Geometry check sheet. Reference: the model listing, model coordinates, mm. Round coordinates to 2 decimals unless told otherwise and drop trailing zeros. Loops run counter-clockwise (first coordinate to the right, second up) from the corner with the lowest first, then second, coordinate; pieces in that order, holes last. Notation, with made-up numbers: M 14.25,74 L 42.25,74 A28 cw 42.25,103 Z; hole C 3,57 d8. An arc over 180 degrees is marked long. Use one line per item in the form item = value. Start each with the question number.
1. Cross-section at C-C (z = 0.1). Record the boundary of the cut face in (x, y), then the cut area to 3 significant figures.
2. Cross-section at A-A (x = 1.5). Record the boundary of the cut face in (y, z).
3. Material ranges on line 1 (X direction, y = 0, z = 0.15); line 2 (X direction, y = 5.25, z = 0.05), recorded low to high.
4. Draft check along X on faces 1 (the flat face through (-7, -2, 0.2)), 2 (the flat face through (2, -7, 0.2)). Enter one of: pulls with the +X half, pulls with the -X half, needs draft (parallel to the pull), parting line crosses it, or undercut.
5. Cross-section at B-B (y = 1). Record the boundary of the cut face in (x, z).
6. Go/stop test with a flat-tipped pin: pin 1 (6 mm diameter, centred on x = 3.5, y = 3.5, fed in from +Z). Record where the tip stops, or that it passes through.
```python
from build123d import *
from build123d.topology import SkipClean

# Parameters (mm, degrees)
SKETCH1_R           = 7.5
SKETCH1_R_2         = 6.75
BOSS_EXTRUDE1_DEPTH = 0.2
BOSS_EXTRUDE3_DEPTH = 0.03


with BuildPart() as part:
    # Sketch1 → Boss-Extrude1 (new body)
    with BuildSketch(Plane.XY):
        Circle(SKETCH1_R)
        Circle(SKETCH1_R_2, mode=Mode.SUBTRACT)
    extrude(amount=BOSS_EXTRUDE1_DEPTH)

    # Sketch2 → Boss-Extrude3 (add)
    with SkipClean():  # the faces are left unmerged after this step: merging them gives an invalid solid
        with BuildSketch(Plane.XY.offset(0.2)):
            with BuildLine():
                Line((3.663064111, 6.544613152), (3.288027069, 5.89502994))
                ThreePointArc((3.288027069, 5.89502994), (3.375, 5.845671476), (3.46123215, 5.79502994))
                Line((3.46123215, 5.79502994), (3.836269192, 6.444613152))
                ThreePointArc((3.836269192, 6.444613152), (3.75, 6.495190528), (3.663064111, 6.544613152))
            make_face()
            with BuildLine():
                Line((-0.1, 7.499333304), (-0.1, 6.749259219))
                ThreePointArc((-0.1, 6.749259219), (0, 6.75), (0.1, 6.749259219))
                Line((0.1, 6.749259219), (0.1, 7.499333304))
                ThreePointArc((0.1, 7.499333304), (0, 7.5), (-0.1, 7.499333304))
            make_face()
            with BuildLine():
                Line((6.444613152, 3.836269192), (5.79502994, 3.46123215))
                ThreePointArc((5.79502994, 3.46123215), (5.845671476, 3.375), (5.89502994, 3.288027069))
                Line((5.89502994, 3.288027069), (6.544613152, 3.663064111))
                ThreePointArc((6.544613152, 3.663064111), (6.495190528, 3.75), (6.444613152, 3.836269192))
            make_face()
            with BuildLine():
                Line((7.499333304, 0.1), (6.749259219, 0.1))
                ThreePointArc((6.749259219, 0.1), (6.75, 0), (6.749259219, -0.1))
                Line((6.749259219, -0.1), (7.499333304, -0.1))
                ThreePointArc((7.499333304, -0.1), (7.5, 0), (7.499333304, 0.1))
            make_face()
            with BuildLine():
                Line((6.544613152, -3.663064111), (5.89502994, -3.288027069))
                ThreePointArc((5.89502994, -3.288027069), (5.845671476, -3.375), (5.79502994, -3.46123215))
                Line((5.79502994, -3.46123215), (6.444613152, -3.836269192))
                ThreePointArc((6.444613152, -3.836269192), (6.495190528, -3.75), (6.544613152, -3.663064111))
            make_face()
            with BuildLine():
                Line((3.836269192, -6.444613152), (3.46123215, -5.79502994))
                ThreePointArc((3.46123215, -5.79502994), (3.375, -5.845671476), (3.288027069, -5.89502994))
                Line((3.288027069, -5.89502994), (3.663064111, -6.544613152))
                ThreePointArc((3.663064111, -6.544613152), (3.75, -6.495190528), (3.836269192, -6.444613152))
            make_face()
            with BuildLine():
                Line((0.1, -7.499333304), (0.1, -6.749259219))
                ThreePointArc((0.1, -6.749259219), (0, -6.75), (-0.1, -6.749259219))
                Line((-0.1, -6.749259219), (-0.1, -7.499333304))
                ThreePointArc((-0.1, -7.499333304), (0, -7.5), (0.1, -7.499333304))
            make_face()
            with BuildLine():
                Line((-3.663064111, -6.544613152), (-3.288027069, -5.89502994))
                ThreePointArc((-3.288027069, -5.89502994), (-3.375, -5.845671476), (-3.46123215, -5.79502994))
                Line((-3.46123215, -5.79502994), (-3.836269192, -6.444613152))
                ThreePointArc((-3.836269192, -6.444613152), (-3.75, -6.495190528), (-3.663064111, -6.544613152))
            make_face()
            with BuildLine():
                Line((-6.444613152, -3.836269192), (-5.79502994, -3.46123215))
                ThreePointArc((-5.79502994, -3.46123215), (-5.845671476, -3.375), (-5.89502994, -3.288027069))
                Line((-5.89502994, -3.288027069), (-6.544613152, -3.663064111))
                ThreePointArc((-6.544613152, -3.663064111), (-6.495190528, -3.75), (-6.444613152, -3.836269192))
            make_face()
            with BuildLine():
                Line((-7.499333304, -0.1), (-6.749259219, -0.1))
                ThreePointArc((-6.749259219, -0.1), (-6.75, 0), (-6.749259219, 0.1))
                Line((-6.749259219, 0.1), (-7.499333304, 0.1))
                ThreePointArc((-7.499333304, 0.1), (-7.5, 0), (-7.499333304, -0.1))
            make_face()
            with BuildLine():
                Line((-6.544613152, 3.663064111), (-5.89502994, 3.288027069))
                ThreePointArc((-5.89502994, 3.288027069), (-5.845671476, 3.375), (-5.79502994, 3.46123215))
                Line((-5.79502994, 3.46123215), (-6.444613152, 3.836269192))
                ThreePointArc((-6.444613152, 3.836269192), (-6.495190528, 3.75), (-6.544613152, 3.663064111))
            make_face()
            with BuildLine():
                Line((-3.836269192, 6.444613152), (-3.46123215, 5.79502994))
                ThreePointArc((-3.46123215, 5.79502994), (-3.375, 5.845671476), (-3.288027069, 5.89502994))
                Line((-3.288027069, 5.89502994), (-3.663064111, 6.544613152))
                ThreePointArc((-3.663064111, 6.544613152), (-3.75, 6.495190528), (-3.836269192, 6.444613152))
            make_face()
        extrude(amount=BOSS_EXTRUDE3_DEPTH)


solid = part.part
```
Reported:
q1.outline = C 0,0 d15; hole C 0,0 d13.5
q1.area = 33.6 mm²
q2.outline = M -7.35,0 L -6.58,0 L -6.58,0.2 L -7.35,0.2 Z; M 6.58,0 L 7.35,0 L 7.35,0.2 L 6.58,0.2 Z
q3.line_1 = -7.5 to -6.75, 6.75 to 7.5
q3.line_2 = -5.36 to -4.24, 4.24 to 5.36
q4.face_1 = needs draft
q4.face_2 = undercut
q5.outline = M -7.43,0 L -6.68,0 L -6.68,0.2 L -7.43,0.2 Z; M 6.68,0 L 7.43,0 L 7.43,0.2 L 6.68,0.2 Z
q6.pin_1 = 0.23
